Could you check a few things on this model? Use its own coordinates, in mm. Round coordinates to 2 decimals unless told otherwise and drop trailing zeros. Order: outer loops, then holes, each group sorted by start corner. A loop starts at its lowest first (then second) coordinate and runs counter-clockwise, first axis right, second up. Notation, with made-up numbers: (11.25, -4) -> (18.25, -4) arc R31 ccw to (18.25, 29) -> close; hole circle Ø10 at (50.5, 71.25). An arc over 180 degrees is marked (long way). Put each result on its own line as item: value. Start each with the question number.
from build123d import *

# Parameters (mm, degrees)
SKETCH_1_R      = 2.6
EXTRUDE_1_DEPTH = 4


with BuildPart() as part:
    # Эскиз1 → Бобышка-Вытянуть1 (new body)
    with BuildSketch(Plane.XY):
        with BuildLine():
            Line((2.5, 0), (77.5, 0))
            ThreePointArc((77.5, 0), (79.267766953, -0.732233047), (80, -2.5))
            Line((80, -2.5), (80, -37.5))
            ThreePointArc((80, -37.5), (79.267766953, -39.267766953), (77.5, -40))
            Line((77.5, -40), (2.5, -40))
            ThreePointArc((2.5, -40), (0.732233047, -39.267766953), (0, -37.5))
            Line((0, -37.5), (0, -2.5))
            ThreePointArc((0, -2.5), (0.732233047, -0.732233047), (2.5, 0))
        make_face()
        with Locations((10, -10)):
            Circle(SKETCH_1_R, mode=Mode.SUBTRACT)
        with Locations((30, -10)):
            Circle(SKETCH_1_R, mode=Mode.SUBTRACT)
        with Locations((50, -10)):
            Circle(SKETCH_1_R, mode=Mode.SUBTRACT)
        with Locations((70, -10)):
            Circle(SKETCH_1_R, mode=Mode.SUBTRACT)
        with Locations((30, -30)):
            Circle(SKETCH_1_R, mode=Mode.SUBTRACT)
        with Locations((50, -30)):
            Circle(SKETCH_1_R, mode=Mode.SUBTRACT)
        with Locations((70, -30)):
            Circle(SKETCH_1_R, mode=Mode.SUBTRACT)
        with Locations((10, -30)):
            Circle(SKETCH_1_R, mode=Mode.SUBTRACT)
    extrude(amount=EXTRUDE_1_DEPTH)


solid = part.part
1. If we section it at C-C, the plane z = 3.25: Count the separate pieces of the cut face and the enclosed holes in it, then the cut area to 3 significant figures.
2. If we section it at A-A, the plane x = 30: Please give me the cut outline in (y, z).
3. For pin 1 Ø8.5 at (x, y) = (50, -30) entering from +Z; pin 2 Ø4 at (x, y) = (50, -10) entering from +Z, each with a flat end and sliding along its axis, tell me the tip position at first contact or that it passes through.
4. I need wall thicknesses on L1, parallel to Y at x = 50, z = 1.05; L2, parallel to Y at x = 68, z = 2.6; L3, parallel to X at y = -12, z = 2.85. Which ranges of each line are inside material? Lowest first, please.
5. If we section it at D-D, the plane x = 50.5: Please give me the cut outline in (y, z), then the cut area to 3 significant figures.
6. If we section it at B-B, the plane y = -30: Please give me the cut outline in (x, z).
7. Thinking about a two-plate mould opening in X: for faces 1 (the face through (0.713, -0.752, 1.972)), 2 (the face through (67.4, -9.9, 2)), 3 (the face through (39, 0, 2)), which applies, +X half, -X half, draft (parallel to the pull), parting line (faces both ways), or undercut?
Results below:
1. separate pieces: 1
1. enclosed holes: 8
1. area: 3,020 mm2
2. outline: (-40, 0) -> (-32.6, 0) -> (-32.6, 4) -> (-40, 4) -> close; (-27.4, 0) -> (-12.6, 0) -> (-12.6, 4) -> (-27.4, 4) -> close; (-7.4, 0) -> (0, 0) -> (0, 4) -> (-7.4, 4) -> close
3. pin 1: z = 4
3. pin 2: through
4. L1: -40 to -32.6, -27.4 to -12.6, -7.4 to 0
4. L2: -40 to -31.66, -28.34 to -11.66, -8.34 to 0
4. L3: 0 to 8.34, 11.66 to 28.34, 31.66 to 48.34, 51.66 to 68.34, 71.66 to 80
5. outline: (-40, 0) -> (-32.55, 0) -> (-32.55, 4) -> (-40, 4) -> close; (-27.45, 0) -> (-12.55, 0) -> (-12.55, 4) -> (-27.45, 4) -> close; (-7.45, 0) -> (0, 0) -> (0, 4) -> (-7.45, 4) -> close
5. area: 119 mm2
6. outline: (0, 0) -> (7.4, 0) -> (7.4, 4) -> (0, 4) -> close; (12.6, 0) -> (27.4, 0) -> (27.4, 4) -> (12.6, 4) -> close; (32.6, 0) -> (47.4, 0) -> (47.4, 4) -> (32.6, 4) -> close; (52.6, 0) -> (67.4, 0) -> (67.4, 4) -> (52.6, 4) -> close; (72.6, 0) -> (80, 0) -> (80, 4) -> (72.6, 4) -> close
7. face 1: -X half
7. face 2: undercut
7. face 3: draft
